Geometry check sheet. Reference: the model listing, model coordinates, mm. Face numbers are marked on the shaded views. A direction names the side the tool comes from. Round coordinates to 2 decimals unless told otherwise and drop trailing zeros. Write each loop counter-clockwise with the first axis right and the second up, starting at its lowest first coordinate (ties: lowest second). Pieces come first, ordered by that corner, then holes.
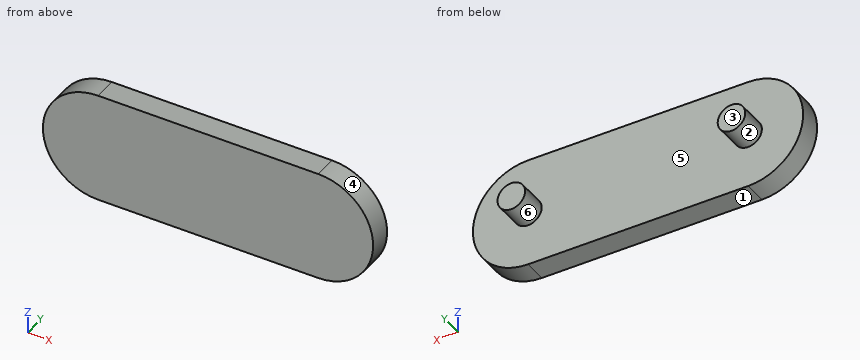
from build123d import *

# Parameters (mm, degrees)
BOSS_EXTRUDE1_DEPTH = 42
SKETCH3_R           = 25
BOSS_EXTRUDE2_DEPTH = 50
SKETCH4_R           = 25
BOSS_EXTRUDE3_DEPTH = 50


with BuildPart() as part:
    # Sketch2 → Boss-Extrude1 (new body)
    with BuildSketch(Plane(origin=(0, 0, 0), x_dir=(1, 0, 0), z_dir=(0, 1, 0))):
        with BuildLine():
            Line((0, -100), (-400, -100))
            ThreePointArc((-400, -100), (-500, 0), (-400, 100))
            Line((-400, 100), (0, 100))
            ThreePointArc((0, 100), (100, 0), (0, -100))
        make_face()
    extrude(amount=BOSS_EXTRUDE1_DEPTH)

    # Sketch3 → Boss-Extrude2 (add)
    with BuildSketch(Plane(origin=(0, 42, 0), x_dir=(1, 0, 0), z_dir=(0, 1, 0))):
        Circle(SKETCH3_R)
    extrude(amount=BOSS_EXTRUDE2_DEPTH)

    # Sketch4 → Boss-Extrude3 (add)
    with BuildSketch(Plane(origin=(0, 42, 0), x_dir=(1, 0, 0), z_dir=(0, 1, 0))):
        with Locations((-400, 0)):
            Circle(SKETCH4_R)
    extrude(amount=BOSS_EXTRUDE3_DEPTH)


solid = part.part
1. Section check A-A (z = 0). Record the cut outline in (x, y), plus the area to 3 significant figures.
2. Access from +Z, -Z, +X, -X, +Y, -Y to the whole of each face (thin tool, end or side, straight path). Record for the marked faces 1 and 2.
3. Release check for a two-part mould opening along X. For the marked faces 3, 4, 5 and 6 record: +X half, -X half, draft (parallel to the pull), parting line (faces both ways), or undercut.
4. Scan lines: line 1 along Y through (x, z) = (-274.5, -46); line 2 along X through (y, z) = (30, -19); line 3 along X through (y, z) = (34, -45). Record each from-to range of solid material in increasing order.
5. Section check C-C (y = 24). Record the cut outline in (x, z), plus the area to 3 significant figures.
6. Section check B-B (y = 49.5). Record the cut outline in (x, z), plus the area to 3 significant figures.
7. Section check D-D (x = -310). Record the cut outline in (y, z), plus the area to 3 significant figures.
8. Depth check by flat-ended pin: pin 1 Ø10 at (x, z) = (-168.5, -14.5) entering from +Y. Enter the tip coordinate at first touch or a pass-through.
Results below:
1. outline: (-500, 0) - (100, 0) - (100, 42) - (25, 42) - (25, 92) - (-25, 92) - (-25, 42) - (-375, 42) - (-375, 92) - (-425, 92) - (-425, 42) - (-500, 42) - close
1. area: 30,200 mm2
2. face 1: -Z, +X, -X, +Y, -Y
2. face 2: +Y
3. face 3: draft
3. face 4: +X half
3. face 5: undercut
3. face 6: undercut
4. line 1: y = 0 to 42
4. line 2: x = -498.18 to 98.18
4. line 3: x = -489.3 to 89.3
5. outline: (-400, -100) - (0, -100) arc R100 ccw to (0, 100) - (-400, 100) arc R100 ccw to start
5. area: 111,000 mm2
6. outline: circle Ø50 at (-400, 0); circle Ø50 at (0, 0)
6. area: 3,930 mm2
7. outline: (0, -100) - (42, -100) - (42, 100) - (0, 100) - close
7. area: 8,400 mm2
8. pin 1: stops at y = 42
